Check sheet for the drawn part. Datum: minimum x, y, z corner. Units: mm. A direction names the side the tool comes from. Give positions to 0.01 mm unless a question says otherwise; leave off trailing zeros. Order: outer loops, then holes, each group sorted by start corner. A loop starts at its lowest first (then second) coordinate and runs counter-clockwise, first axis right, second up. Notation, with made-up numbers: M 86,33 L 125,33 A33 ccw 125,69 Z; hole C 71.25,54 d5. An arc over 180 degrees is marked long. Put each result on its own line as item: value. Start each with the question number.
Q1. Section check D-D on z = 9.5. Record the cut outline in (x, y).
Q2. Section check B-B on x = 22.5. Record the cut outline in (y, z) (1 decimal).
Q3. Mould release check, pull along Y, two halves, no side actions. Record for the marked faces 4, 5, 6 and 7: +Y half, -Y half, draft (parallel to the pull), parting line (faces both ways), or undercut.
Q4. Access from +Z, -Z, +X, -X, +Y, -Y to the whole of each face (thin tool, end or side, straight path). Record for the marked faces 1, 2 and 3.
Q5. Section check A-A on z = 17.5. Record the cut outline in (x, y) (1 decimal).
Q6. Section check C-C on y = 7. Record the cut outline in (x, z) (1 decimal).
Q7. Go/stop test with flat-tipped pins: pin 1 (7 mm diameter, centred on x = 20.5, y = 7.5, fed in from +Z); pin 2 (7 mm diameter, centred on x = 14.5, z = 1.5, fed in from -Y); pin 3 (1.5 mm diameter, centred on x = 7, z = 11.5, fed in from +Y) (1 decimal). Record where each tip stops, or that it passes through.
Q8. Material ranges on L1, parallel to X at y = 34.5, z = 9.75; L2, parallel to Z at x = 11, y = 16; L3, parallel to Y at x = 44.5, z = 17 (1 decimal), recorded low to high.
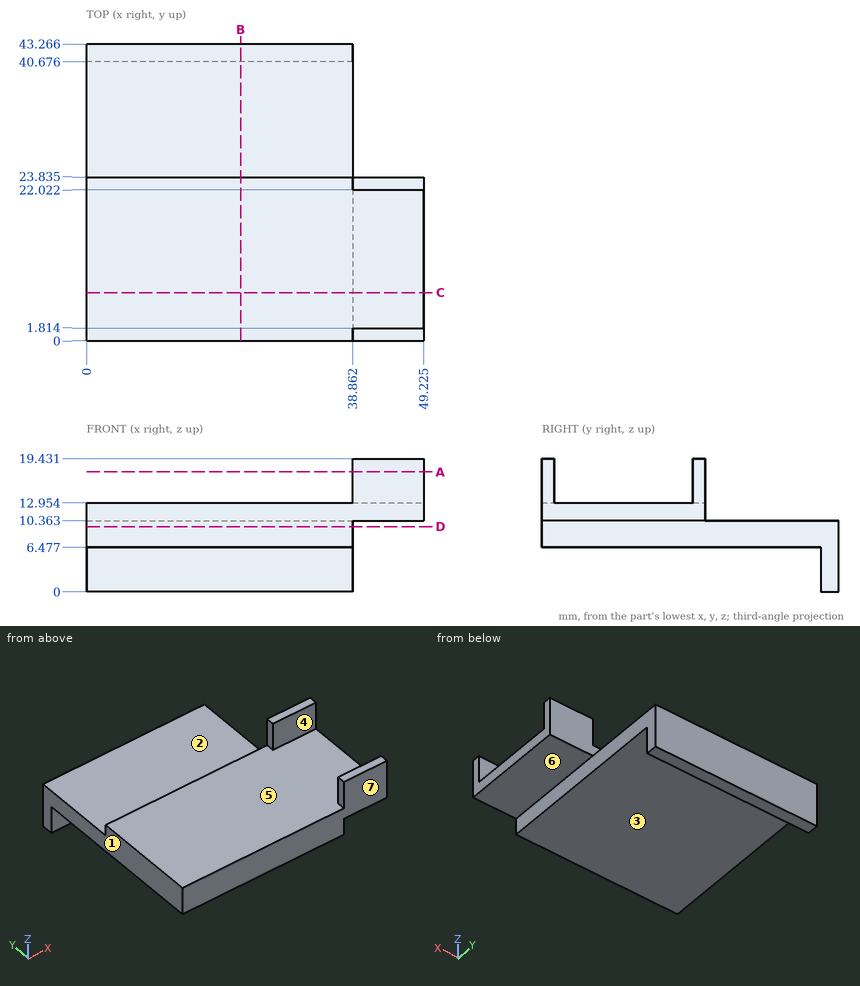
Results found:
1. outline: M 0,0 L 38.86,0 L 38.86,43.27 L 0,43.27 Z
2. outline: M 0,6.5 L 40.7,6.5 L 40.7,0 L 43.3,0 L 43.3,10.4 L 23.8,10.4 L 23.8,13 L 0,13 Z
3. face 4: undercut
3. face 5: undercut
3. face 6: draft
3. face 7: -Y half
4. face 1: +Z, -Z, -X, +Y, -Y
4. face 2: +Z, +X, -X, +Y
4. face 3: -Z, +X, -X, -Y
5. outline: M 38.9,0 L 49.2,0 L 49.2,1.8 L 38.9,1.8 Z; M 38.9,22 L 49.2,22 L 49.2,23.8 L 38.9,23.8 Z
6. outline: M 0,6.5 L 38.9,6.5 L 38.9,10.4 L 49.2,10.4 L 49.2,13 L 0,13 Z
7. pin 1: stops at z = 12.95
7. pin 2: stops at y = 40.68
7. pin 3: stops at y = 23.8
8. L1: x = 0 to 38.86
8. L2: z = 6.48 to 12.95
8. L3: y = 0 to 1.8, 22 to 23.8
